Check sheet for the modelled part. Datum: model origin and axes. Units: mm. A direction names the side the tool comes from. Round coordinates to 2 decimals unless told otherwise and drop trailing zeros. Loops run counter-clockwise (first coordinate to the right, second up) from the corner with the lowest first, then second, coordinate; pieces in that order, holes last. Notation, with made-up numbers: (36.25, 39.5) - (88.25, 39.5) arc R19 cw to (88.25, 71.5) - close; hole circle Ø8 at (25, -1.5). An arc over 180 degrees is marked (long way). Put each result on its own line as item: value. Start each with the question number.
Item 1: Tool access check on faces 5 (the flat face through (55, 13.97, 4)), 6 (the flat face through (17.4, -13.3, 0)). Record the directions out of +Z, -Z, +X, -X, +Y, -Y that give a thin tool (end or side, any length) a straight path to the whole face; none if there is none.
Item 2: Section check A-A, the plane y = 0. Record the cut outline in (x, z), and give its area (3 significant figures).
Item 3: Material ranges on line 1 along X through (y, z) = (0.5, 1.5); line 2 along Y through (x, z) = (0, 3.75); line 3 along Y through (x, z) = (54, 3), recorded low to high.
Item 4: Section check B-B, the plane x = 0. Record the cut outline in (y, z).
Item 5: Gauge pin test, flat ends, axial feed: pin 1 Ø2.5 at (x, y) = (24.98, -9.48) entering from +Z; pin 2 Ø2.5 at (x, z) = (-52, 4) entering from +Y. Record the tip position at first contact, or that the pin passes through.
Item 6: Draft check along Y on faces 1 (the flat face through (17.4, -13.3, 7.62)), 2 (the flat face through (-55, 13.97, 4)), 3 (the cylindrical face through (26.075, -7.771, 3.863)), 4 (the cylindrical face through (-26.4, -18.82, 3.86)). Enter one of: pulls with the +Y half, pulls with the -Y half, needs draft (parallel to the pull), parting line crosses it, or undercut.
Item 7: Section check C-C, the plane z = 4. Record the cut outline in (x, y).
Item 8: Section check D-D, the plane x = -34. Record the cut outline in (y, z), and give its area (3 significant figures).
from build123d import *

# Parameters (mm, degrees)
SKETCH1_R           = 38.1
SKETCH1_R_2         = 21.59
BOSS_EXTRUDE1_DEPTH = 7.62
CUT_EXTRUDE1_DEPTH  = 55.417684625
SKETCH7_R           = 2.032
CUT_EXTRUDE2_DEPTH  = 55.417684625
BOSS_EXTRUDE2_START = -7.62
BOSS_EXTRUDE2_DEPTH = 7.62


with BuildPart() as part:
    # Sketch1 → Boss-Extrude1 (new body)
    with BuildSketch(Plane.XY):
        with Locations(Location((0, 0, 0), (0, 0, 180))):
            Circle(SKETCH1_R)
        with Locations(Location((0, 0, 0), (0, 0, 180))):
            Circle(SKETCH1_R_2, mode=Mode.SUBTRACT)
    extrude(amount=BOSS_EXTRUDE1_DEPTH)

    # Sketch2 → Cut-Extrude1 (cut, through all)
    with BuildSketch(Plane.XY.offset(7.62)):
        Polygon((0, -38.1), (-36.256055522, -38.1), (-36.256055522, -24.13), (33.75035888, -24.13), (33.75035888, -38.1), align=None)
    extrude(amount=-CUT_EXTRUDE1_DEPTH, mode=Mode.SUBTRACT)

    # Sketch7 → Cut-Extrude2 (cut, through all)
    with BuildSketch(Plane.XY.offset(7.62)):
        with Locations((-24.902829883, -20.191092866)):
            Circle(SKETCH7_R)
        with Locations((-5.581705562, 30.037407134)):
            Circle(SKETCH7_R)
        with Locations((24.982770117, -9.484666265)):
            Circle(SKETCH7_R)
    extrude(amount=-CUT_EXTRUDE2_DEPTH, mode=Mode.SUBTRACT)

    # Sketch9 → Boss-Extrude2 (add)
    with BuildSketch(Plane.XY.offset(7.62).offset(BOSS_EXTRUDE2_START)):
        Polygon((-29.484794386, -24.13), (-73.546425772, -24.13), (-73.546425772, 13.97), (-35.446425772, 13.97), align=None)
        Polygon((29.484794386, -24.13), (73.546425772, -24.13), (73.546425772, 13.97), (35.446425772, 13.97), align=None)
    extrude(amount=BOSS_EXTRUDE2_DEPTH)


solid = part.part
Check result:
1. face 5: +Z, -Z, +X, +Y
1. face 6: -Z, +X, -X, +Y, -Y
2. outline: (-73.55, 0) - (-21.59, 0) - (-21.59, 7.62) - (-73.55, 7.62) - close; (21.59, 0) - (73.55, 0) - (73.55, 7.62) - (21.59, 7.62) - close
2. area: 792 mm²
3. line 1: -73.55 to -21.58, 21.58 to 73.55
3. line 2: -24.13 to -21.59, 21.59 to 38.1
3. line 3: -24.13 to 13.97
4. outline: (-24.13, 0) - (-21.59, 0) - (-21.59, 7.62) - (-24.13, 7.62) - close; (21.59, 0) - (38.1, 0) - (38.1, 7.62) - (21.59, 7.62) - close
5. pin 1: through
5. pin 2: y = 13.97
6. face 1: needs draft
6. face 2: pulls with the +Y half
6. face 3: undercut
6. face 4: undercut
7. outline: (-73.55, -24.13) - (73.55, -24.13) - (73.55, 13.97) - (35.45, 13.97) arc R38.1 ccw to (-35.45, 13.97) - (-73.55, 13.97) - close; hole circle Ø4.06 at (-24.9, -20.19); hole circle Ø43.18 at (0, 0); hole circle Ø4.06 at (-5.58, 30.04); hole circle Ø4.06 at (24.98, -9.48)
8. outline: (-24.13, 0) - (17.19, 0) - (17.19, 7.62) - (-24.13, 7.62) - close
8. area: 315 mm²
